Source: CAD feature listing. Evaluate the final solid. Frame: model axes, mm. Face numbers are marked on the shaded views. A direction names the side the tool comes from. Give positions to 0.01 mm unless a question says otherwise; leave off trailing zeros. Loops run counter-clockwise (first coordinate to the right, second up) from the corner with the lowest first, then second, coordinate; pieces in that order, holes last. Notation, with made-up numbers: (39.25, -14) - (93.25, -14) arc R18 cw to (93.25, 11) - close; hole circle Ø9 at (-28.5, -30). An arc over 180 degrees is marked (long way). Write each question's results on one line, items separated by ' | '. Start each with the question number.
(1) Cut plane D-D on x = -36.5. Return the cut outline in (y, z), then the cut area to 3 significant figures.
(2) Material intervals for line 1 along Y through (x, z) = (-41, 11); line 2 along Y through (x, z) = (-36, 2.75); line 3 along Y through (x, z) = (-34, 7.5), sorted ascending. Write a range as [from, to].
(3) Cut plane B-B on x = -8. Return the cut outline in (y, z).
(4) Cut plane A-A on y = 0. Return the cut outline in (x, z).
(5) Pull-direction query (Y, two-part tool) for the marked faces 1, 2 and 3; classes: pulls with the +Y half, pulls with the -Y half, needs draft (parallel to the pull), parting line crosses it, or undercut.
(6) Contact query for flat-ended pins moving along their axis: pin 1 (1 mm diameter, centred on x = -25, z = 7.5, fed in from -Y); pin 2 (8 mm diameter, centred on y = -33, z = 5.5, fed in from +X); pin 3 (4 mm diameter, centred on y = -23.5, z = 10.5, fed in from +X). Output: stop coordinate, or through.
(7) Reachability of the marked faces 4, 5 and 6 from +Z, -Z, +X, -X, +Y, -Y: full face, straight path, thin tool, end or side. Return the list, or none.
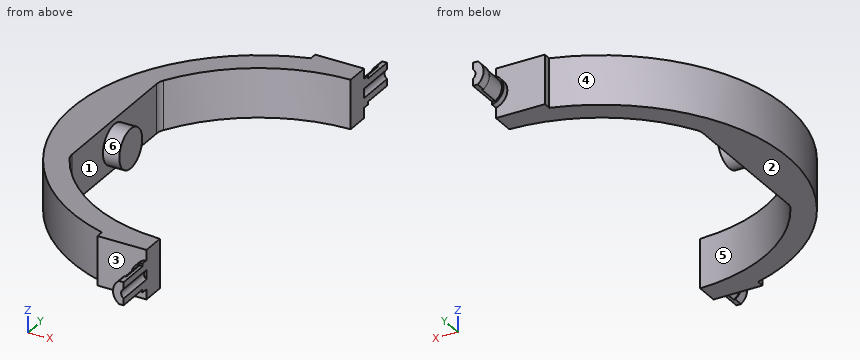
from build123d import *

# Parameters (mm, degrees)
F1_DEPTH  = 15
F2_R      = 6
F3_DEPTH  = 5
F4_R      = 5
F6_DEPTH  = 2
F8_DEPTH  = 7
F10_DEPTH = 3
F11_DEPTH = 25
F13_W     = 146.8421146274
F13_H     = 28.1250011176
F14_DEPTH = 1
F15_W     = 11.3657170441
F15_H     = 11.5304403007
F15_W_2   = 13.3423628286
F15_H_2   = 13.0129233003
F16_DEPTH = 4
F17_W     = 19.5150814822
F17_H     = 12.7272193491
F17_W_2   = 18.9494257321
F17_H_2   = 10.7474377315
F18_DEPTH = 4


with BuildPart() as f1:
    # F0 (on Top) → F1 (new body)
    with BuildSketch(Plane.XY):
        with BuildLine():
            ThreePointArc((-44.16, 23.4498272915), (-25.7634298515, 42.8514373421), (0, 50))
            Line((0, 50), (0, 57))
            Line((0, 57), (-15.9976914198, 57))
            Line((-15.9976914198, 57), (-15.9976914198, 54.7089925811))
            ThreePointArc((-15.9976914198, 54.7089925811), (-57, 0), (-15.9976914198, -54.7089925811))
            Line((-15.9976914198, -54.7089925811), (-15.9976914198, -57))
            Line((-15.9976914198, -57), (0, -57))
            Line((0, -57), (0, -50))
            ThreePointArc((0, -50), (-25.7634298515, -42.8514373421), (-44.16, -23.4498272915))
            Line((-44.16, -23.4498272915), (-44.16, 23.4498272915))
        make_face()
    extrude(amount=F1_DEPTH)

    # F2 (on face) → F3 (join)
    with BuildSketch(Plane.YZ.offset(-44.16)):
        with Locations((0, 7.5)):
            Circle(F2_R)
    extrude(amount=F3_DEPTH)

    # F4
    f4_edges = [f1.edges().sort_by_distance(p)[0] for p in [
        (-44.16, 23.449827, 7.5),
        (-44.16, -23.449827, 7.5),
    ]]
    fillet(f4_edges, radius=F4_R)

    # F5 (on face) → F6 (join)
    with BuildSketch(Plane.XZ.offset(57)):
        with BuildLine():
            Line((0, 9.25), (0, 12))
            ThreePointArc((0, 12), (-4.5, 7.5), (0, 3))
            Line((0, 3), (0, 5.75))
            ThreePointArc((0, 5.75), (-1.75, 7.5), (0, 9.25))
        make_face()
    extrude(amount=F6_DEPTH)

    # F7 (on face) → F8 (join)
    with BuildSketch(Plane.XZ.offset(59)):
        with BuildLine():
            Line((0, 9.25), (0, 11.5))
            ThreePointArc((0, 11.5), (-4, 7.5), (0, 3.5))
            Line((0, 3.5), (0, 5.75))
            ThreePointArc((0, 5.75), (-1.75, 7.5), (0, 9.25))
        make_face()
    extrude(amount=F8_DEPTH)

    # F9 (on face) → F10 (join)
    with BuildSketch(Plane.XZ.offset(66)):
        with BuildLine():
            Line((0, 3.25), (0, 11.75))
            ThreePointArc((0, 11.75), (-4.25, 7.5), (0, 3.25))
        make_face()
    extrude(amount=F10_DEPTH)

    # F11 (cut): a face of the model
    f11_faces = [f1.faces().sort_by_distance(p)[0] for p in [
        (-0.7427230678, -66, 7.5),
    ]]
    extrude(f11_faces, amount=-F11_DEPTH, mode=Mode.SUBTRACT)

    # F12: F1 across plane


with BuildPart() as f1_1:
    add(f1.part)
    add(f1.part.mirror(Plane.XZ))

    # F13 (on Right) → F14 (cut)
    with BuildSketch(Plane.YZ):
        with Locations((0.2960525453, 7.5493426993)):
            Rectangle(F13_W, F13_H)
    extrude(amount=-F14_DEPTH, mode=Mode.SUBTRACT)

    # F15 (on Top) → F16 (cut)
    with BuildSketch(Plane.XY):
        with Locations((-1.9552764716, -64.7652201504)):
            Rectangle(F15_W, F15_H)
        with Locations((-2.1199961193, 65.5064616501)):
            Rectangle(F15_W_2, F15_H_2)
    extrude(amount=F16_DEPTH, mode=Mode.SUBTRACT)

    # F17 (on face) → F18 (cut)
    with BuildSketch(Plane.XY.offset(15)):
        with Locations((-4.4578294758, 65.3636096745)):
            Rectangle(F17_W, F17_H)
        with Locations((-2.7608656596, -64.3737188657)):
            Rectangle(F17_W_2, F17_H_2)
    extrude(amount=-F18_DEPTH, mode=Mode.SUBTRACT)


solid = f1_1.part
Ans:
1) outline: (-43.78, 0) - (-34.17, 0) - (-34.17, 15) - (-43.78, 15) - close; (34.17, 0) - (43.78, 0) - (43.78, 15) - (34.17, 15) - close | area: 288 mm^2
2) line 1: [-39.6, -28.62], [-4.87, 4.87], [28.62, 39.6] | line 2: [-44.19, -34.7], [34.7, 44.19] | line 3: [-45.75, -36.66], [36.66, 45.75]
3) outline: (-57, 0) - (-49.36, 0) - (-49.36, 15) - (-57, 15) - close; (49.36, 0) - (57, 0) - (57, 15) - (49.36, 15) - close
4) outline: (-57, 0) - (-44.16, 0) - (-44.16, 1.5) - (-39.16, 1.5) - (-39.16, 13.5) - (-44.16, 13.5) - (-44.16, 15) - (-57, 15) - close
5) face 1: undercut | face 2: needs draft | face 3: pulls with the -Y half
6) pin 1: y = -51.47 | pin 2: x = -33.63 | pin 3: x = -43.01
7) face 4: +Z, -Z, -X | face 5: +Z, -Z, +X | face 6: +X
